```python
from build123d import *

# Parameters (mm, degrees)
F1_DEPTH = 60
F2_R     = 29.99999
F3_R     = 15
F4_DEPTH = 25
F5_R     = 5
F6_W     = 46
F6_H     = 16
F7_DEPTH = 25
F6_R     = 2.5
F8_DEPTH = 25
F9_R     = 7.99999


# Not quite as in the source:
# - a fillet or chamfer is up to 0.001 mm smaller than in the source, because OpenCascade refuses the exact size


with BuildPart() as f1:
    # F0 (on Front) → F1 (new body)
    with BuildSketch(Plane.XZ):
        Polygon((80, 0), (0, 0), (0, -10), (77.3205080757, -10), align=None)
        Polygon((131.9615242271, -30), (80, 0), (77.3205080757, -10), (126.9615242271, -38.6602540378), align=None)
    extrude(amount=F1_DEPTH)

    # F2 (radius 30 in the source; OpenCascade refuses exactly that, so slightly less here)
    f2_edges = [f1.edges().sort_by_distance(p)[0] for p in [
        (129.461524, 0, -34.330127),
        (129.461524, -60, -34.330127),
    ]]
    fillet(f2_edges, radius=F2_R)

    # F3 (on face) → F4 (cut)
    with BuildSketch(Plane(origin=(20, 0, 34.6410161514), x_dir=(0.8660254038, 0, -0.5), z_dir=(0.5, 0, 0.8660254038))):
        with Locations((99.2820323028, -30)):
            Circle(F3_R)
    extrude(amount=-F4_DEPTH, mode=Mode.SUBTRACT)

    # F5
    f5_edges = [f1.edges().sort_by_distance(p)[0] for p in [
        (0, 0, -5),
        (0, -60, -5),
    ]]
    fillet(f5_edges, radius=F5_R)

    # F6 (on face) → F7 (cut)
    with BuildSketch(Plane.XY):
        with Locations((40, -30)):
            Rectangle(F6_W, F6_H)
    extrude(amount=-F7_DEPTH, mode=Mode.SUBTRACT)

    # F6 (on face) → F8 (cut)
    with BuildSketch(Plane.XY):
        with Locations((10, -50)):
            Circle(F6_R)
        with Locations((70, -50)):
            Circle(F6_R)
        with Locations((70, -10)):
            Circle(F6_R)
        with Locations((10, -10)):
            Circle(F6_R)
        with Locations((40, -30)):
            Rectangle(F6_W, F6_H)
    extrude(amount=-F8_DEPTH, mode=Mode.SUBTRACT)

    # F9 (radius 8 in the source; OpenCascade refuses exactly that, so slightly less here)
    f9_edges = [f1.edges().sort_by_distance(p)[0] for p in [
        (63, -22, -5),
        (63, -38, -5),
        (17, -22, -5),
        (17, -38, -5),
    ]]
    fillet(f9_edges, radius=F9_R)


solid = f1.part
```
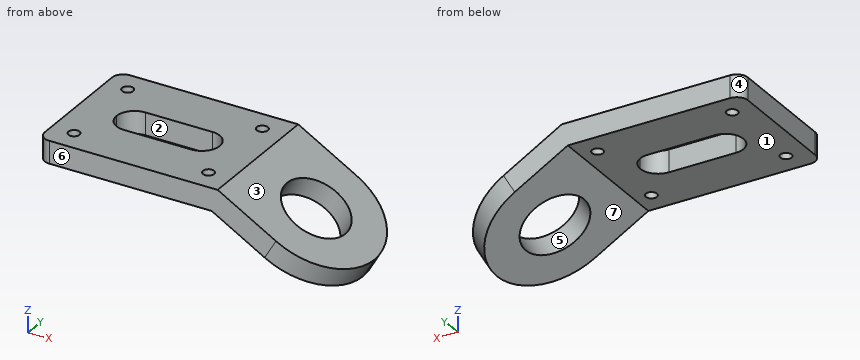
Read the model definition and answer for the solid it produces. Units are mm, in the model's axes. Face numbers are marked on the shaded views. A direction names the side the tool comes from. Give positions to 0.01 mm unless a question says otherwise; leave off trailing zeros. Order: outer loops, then holes, each group sorted by start corner. A loop starts at its lowest first (then second) coordinate and runs counter-clockwise, first axis right, second up. Notation, with made-up numbers: (79.25, 56.25) -> (114.25, 56.25) arc R16 ccw to (114.25, 68.25) -> close; hole circle Ø5 at (53.25, 55.25). An arc over 180 degrees is marked (long way). One line per item, written item: value. Start each with the question number.
(1) The part is cut by section B-B (x = 33). Determine the outline of the cut face in (y, z), and give its area (3 significant figures).
(2) Straight lines are drawn through the part: L1, parallel to Y at x = 70, z = -3; L2, parallel to Y at x = 44.5, z = -9; L3, parallel to Z at x = 8, y = -52. For each, find the intervals that lie inside material, in ascending order.
(3) The part is cut by section A-A (x = 70). Determine the outline of the cut face in (y, z).
(4) Flat-ended cylindrical pins translate along their axes: P1, Ø6, axis at y = -28.5, z = -20, coming from the -X side; P2, Ø2, axis at x = 31.5, y = -22.5, coming from the -Z side; P3, Ø5, axis at y = -10, z = -27, coming from the +X side; P4, Ø3, axis at x = 70, y = -10, coming from the +Z side. Find the tip coordinate at first contact, or state that the pin passes through.
(5) The part is cut by section C-C (y = -35.5). Determine the outline of the cut face in (x, z).
(6) A tool of negligible diameter and unlimited length cuts with its end or side. For the marked faces 1, 2 and 3, from which of +Z, -Z, +X, -X, +Y, -Y can it reach the whole face along a straight path? Write none if from no direction.
(7) For a pull along Y with two mould halves and no side action, classify the marked faces 4, 5, 6 and 7 as released by +Y, released by -Y, zero draft, split by the parting line, or undercut.
(8) The part is cut by section D-D (z = -3). State how many separate pieces and enclosed holes the cut face has, and give its area (3 significant figures).
Taken from the geometry:
1. outline: (-60, -10) -> (-38, -10) -> (-38, 0) -> (-60, 0) -> close; (-22, -10) -> (0, -10) -> (0, 0) -> (-22, 0) -> close
1. area: 440 mm^2
2. L1: -60 to -52.5, -47.5 to -12.5, -7.5 to 0
2. L2: -60 to -38, -22 to 0
2. L3: -10 to 0
3. outline: (-60, -10) -> (-52.5, -10) -> (-52.5, 0) -> (-60, 0) -> close; (-47.5, -10) -> (-12.5, -10) -> (-12.5, 0) -> (-47.5, 0) -> close; (-7.5, -10) -> (0, -10) -> (0, 0) -> (-7.5, 0) -> close
4. P1: x = 118.54
4. P2: z = -10
4. P3: x = 127.08
4. P4: through
5. outline: (0, -10) -> (19.19, -10) -> (19.19, 0) -> (0, 0) -> close; (60.81, -10) -> (77.32, -10) -> (88.9, -16.68) -> (93.9, -8.02) -> (80, 0) -> (60.81, 0) -> close; (113.07, -30.64) -> (126.52, -38.41) -> (131.52, -29.75) -> (118.07, -21.98) -> close
6. face 1: -Z, -X, +Y, -Y
6. face 2: +Z, -Z
6. face 3: +Z, +X, +Y, -Y
7. face 4: released by +Y
7. face 5: undercut
7. face 6: released by -Y
7. face 7: zero draft
8. separate pieces: 1
8. enclosed holes: 5
8. area: 4,340 mm^2
